Design review of the part built by this model. Coordinates are the model's own, in mm. Face numbers are marked on the shaded views. A direction names the side the tool comes from. Coordinates: 2 decimals unless noted, no trailing zeros. Loops run counter-clockwise (first coordinate to the right, second up) from the corner with the lowest first, then second, coordinate; pieces in that order, holes last. Notation, with made-up numbers: (23, -8) -> (54, -8) arc R24 cw to (54, 3) -> close; hole circle Ø5 at (-38.5, -5.5). An arc over 180 degrees is marked (long way). Use one line per item in the form item = value. Start each with the question number.
1. Machinability: for the marked faces 1, 2, 3 and 4, which of the approach directions +Z, -Z, +X, -X, +Y, -Y give a long, thin tool a straight path to every point of the face, cutting with its end or side? Answer none if there is none.
2. Wall thickness on line 1 (Y direction, x = 1, z = 2.5); line 2 (Z direction, x = 4.5, y = 1.5); line 3 (Z direction, x = -1.5, y = -0.6): over which ranges is each line inside the solid? List them lowest first. Write a range as from..to.
3. Consider section A-A (x = 0.75). State the section outline as (y, z) points, then the cut area to 3 significant figures.
4. For pin 1 (1 mm diameter, centred on x = 1.5, z = 2, fed in from +Y); pin 2 (2 mm diameter, centred on x = 1, z = 2, fed in from -Y); pin 3 (2 mm diameter, centred on x = -2, z = 0.5, fed in from +Y); pin 4 (1 mm diameter, centred on x = 1.5, y = 1, fed in from -Z), all flat-tipped, find the tip position at first contact; note any pin that passes through.
5. Consider section D-D (x = 2.5). State the section outline as (y, z) points.
6. Consider section C-C (z = 0.25). State the section outline as (x, y) points, then the cut area to 3 significant figures.
7. Consider section B-B (y = 0). State the section outline as (x, z) points, then the cut area to 3 significant figures.
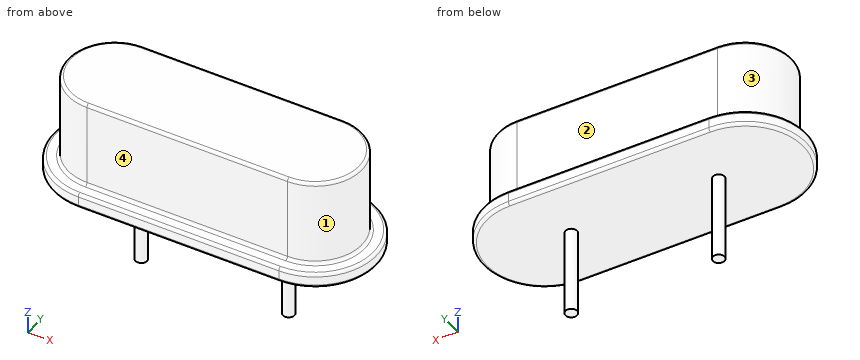
from build123d import *

# Parameters (mm, degrees)
EXTRUDE_1_DEPTH = 0.5
EXTRUDE_2_DEPTH = 3
SKETCH_3_R      = 0.2
EXTRUDE_3_DEPTH = 3
FILLET_1_R      = 0.1


with BuildPart() as part:
    # 草图1 → 凸台-拉伸1 (new body)
    with BuildSketch(Plane.XY):
        with BuildLine():
            Line((3.4, 2.1), (-3.4, 2.1))
            ThreePointArc((-3.4, 2.1), (-5.5, 0), (-3.4, -2.1))
            Line((-3.4, -2.1), (3.4, -2.1))
            ThreePointArc((3.4, -2.1), (5.5, 0), (3.4, 2.1))
        make_face()
    extrude(amount=EXTRUDE_1_DEPTH)

    # 草图2 → 凸台-拉伸2 (add)
    with BuildSketch(Plane.XY.offset(0.5)):
        with BuildLine():
            Line((-3.4, 1.6), (3.4, 1.6))
            ThreePointArc((3.4, 1.6), (5, 0), (3.4, -1.6))
            Line((3.4, -1.6), (-3.4, -1.6))
            ThreePointArc((-3.4, -1.6), (-5, 0), (-3.4, 1.6))
        make_face()
    extrude(amount=EXTRUDE_2_DEPTH)

    # 草图3 → 凸台-拉伸3 (add)
    with BuildSketch(Plane(origin=(0, 0, 0), x_dir=(-1, 0, 0), z_dir=(0, 0, -1))):
        with Locations(Location((-2.5, 0, 0), (0, 0, 180))):
            Circle(SKETCH_3_R)
        with Locations(Location((2.5, 0, 0), (0, 0, 180))):
            Circle(SKETCH_3_R)
    extrude(amount=EXTRUDE_3_DEPTH)

    # 圆角1
    fillet_1_edges = [part.edges().sort_by_distance(p)[0] for p in [
        (-5.5, 0, 0.5),
        (0, -2.1, 0.5),
        (5, 0, 0.5),
        (0, 1.6, 0.5),
        (-5, 0, 0.5),
        (0, -1.6, 0.5),
        (5, 0, 3.5),
        (0, 1.6, 3.5),
        (-5, 0, 3.5),
        (0, -1.6, 3.5),
        (5.5, 0, 0.5),
        (0, -2.1, 0),
        (-5.5, 0, 0),
        (0, 2.1, 0),
        (5.5, 0, 0),
        (0, 2.1, 0.5),
    ]]
    fillet(fillet_1_edges, radius=FILLET_1_R)


solid = part.part
Geometry check:
q1.face_1 = +Z, +X
q1.face_2 = +Z, +X, -X, +Y
q1.face_3 = +Z, -X
q1.face_4 = +Z, +X, -X, -Y
q2.line_1 = -1.6..1.6
q2.line_2 = 0..0.5
q2.line_3 = 0..3.5
q3.outline = (-2.1, 0.1) arc R0.1 ccw to (-2, 0) -> (2, 0) arc R0.1 ccw to (2.1, 0.1) -> (2.1, 0.4) arc R0.1 ccw to (2, 0.5) -> (1.7, 0.5) arc R0.1 cw to (1.6, 0.6) -> (1.6, 3.4) arc R0.1 ccw to (1.5, 3.5) -> (-1.5, 3.5) arc R0.1 ccw to (-1.6, 3.4) -> (-1.6, 0.6) arc R0.1 cw to (-1.7, 0.5) -> (-2, 0.5) arc R0.1 ccw to (-2.1, 0.4) -> close
q3.area = 11.7 mm²
q4.pin_1 = 1.6
q4.pin_2 = -1.6
q4.pin_3 = 2.1
q4.pin_4 = 0
q5.outline = (-2.1, 0.1) arc R0.1 ccw to (-2, 0) -> (-0.2, 0) -> (-0.2, -3) -> (0.2, -3) -> (0.2, 0) -> (2, 0) arc R0.1 ccw to (2.1, 0.1) -> (2.1, 0.4) arc R0.1 ccw to (2, 0.5) -> (1.7, 0.5) arc R0.1 cw to (1.6, 0.6) -> (1.6, 3.4) arc R0.1 ccw to (1.5, 3.5) -> (-1.5, 3.5) arc R0.1 ccw to (-1.6, 3.4) -> (-1.6, 0.6) arc R0.1 cw to (-1.7, 0.5) -> (-2, 0.5) arc R0.1 ccw to (-2.1, 0.4) -> close
q6.outline = (-3.4, -2.1) -> (3.4, -2.1) arc R2.1 ccw to (3.4, 2.1) -> (-3.4, 2.1) arc R2.1 ccw to start
q6.area = 42.4 mm²
q7.outline = (-5.5, 0.1) arc R0.1 ccw to (-5.4, 0) -> (-2.7, 0) -> (-2.7, -3) -> (-2.3, -3) -> (-2.3, 0) -> (2.3, 0) -> (2.3, -3) -> (2.7, -3) -> (2.7, 0) -> (5.4, 0) arc R0.1 ccw to (5.5, 0.1) -> (5.5, 0.4) arc R0.1 ccw to (5.4, 0.5) -> (5.1, 0.5) arc R0.1 cw to (5, 0.6) -> (5, 3.4) arc R0.1 ccw to (4.9, 3.5) -> (-4.9, 3.5) arc R0.1 ccw to (-5, 3.4) -> (-5, 0.6) arc R0.1 cw to (-5.1, 0.5) -> (-5.4, 0.5) arc R0.1 ccw to (-5.5, 0.4) -> close
q7.area = 37.9 mm²
